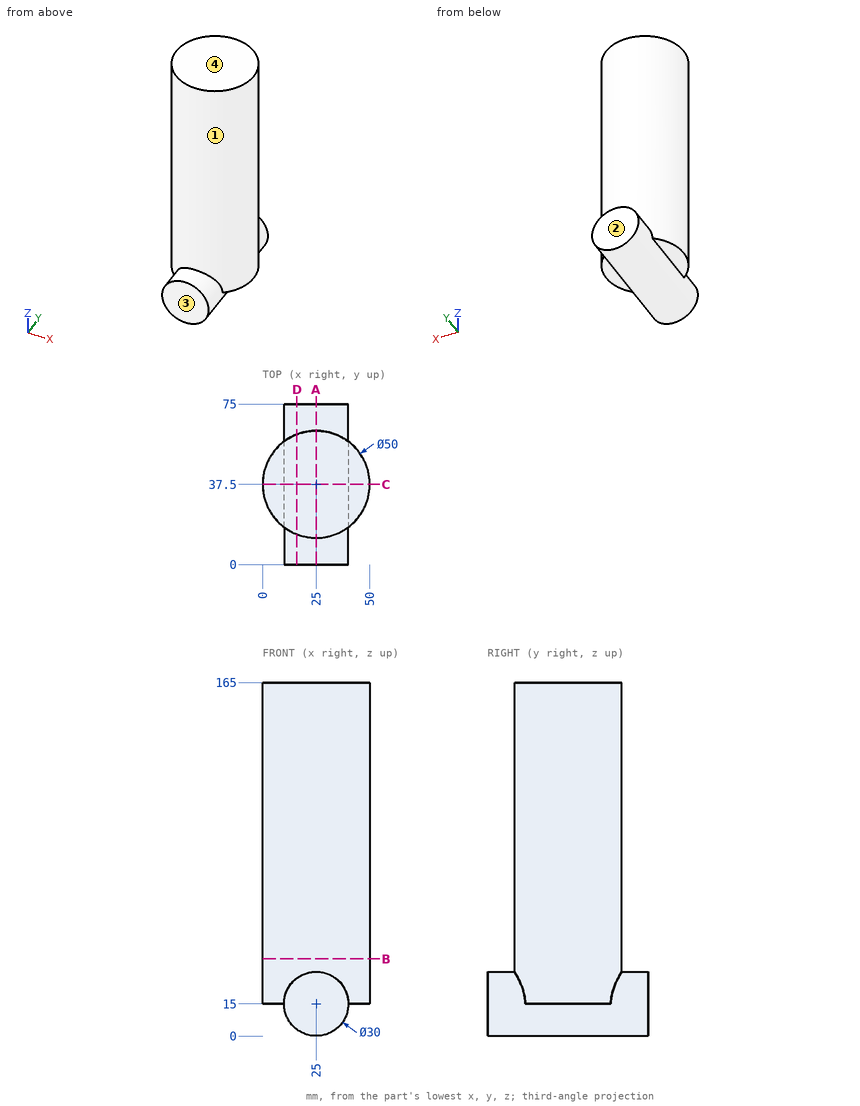
Here's the drawing with two shaded views (mm, measured from the low corner). I have some questions. Coordinates: 2 decimals unless noted, no trailing zeros. Order: outer loops, then holes, each group sorted by start corner. A loop starts at its lowest first (then second) coordinate and runs counter-clockwise, first axis right, second up.
Item 1: If we section it at A-A on x = 25: List the corners of the cut face in (y, z) for me.
Result sheet:
outline: (0, 0) - (75, 0) - (75, 30) - (62.5, 30) - (62.5, 165) - (12.5, 165) - (12.5, 30) - (0, 30) - close
Item 2: If we section it at D-D on x = 16: List the corners of the cut face in (y, z) for me, plus the area to 3 significant figures.
Result sheet:
outline: (0, 3) - (75, 3) - (75, 27) - (60.82, 27) - (60.82, 165) - (14.18, 165) - (14.18, 27) - (0, 27) - close
area: 8,240 mm2
Item 3: If we mould it in two halves opening along Y, with no side actions, what happens to the marked faces 1, 2, 3 and 4? For each: +Y half, -Y half, draft (parallel to the pull), parting line (faces both ways), or undercut.
Result sheet:
face 1: parting line
face 2: +Y half
face 3: -Y half
face 4: draft
Item 4: I need wall thicknesses on line 1 (Z direction, x = 26, y = 21.5); line 2 (Z direction, x = 26, y = 72); line 3 (Y direction, x = 33, z = 80). Which ranges of each line are inside material? Lowest first, please.
Result sheet:
line 1: z = 0.03 to 165
line 2: z = 0.03 to 29.97
line 3: y = 13.81 to 61.19
Item 5: If we section it at B-B on z = 36: List the corners of the cut face in (x, y) for me.
Result sheet:
outline: circle Ø50 at (25, 37.5)
Item 6: If we section it at C-C on y = 37.5: List the corners of the cut face in (x, z) for me, plus the area to 3 significant figures.
Result sheet:
outline: (0, 15) - (10, 15) arc R15 ccw to (40, 15) - (50, 15) - (50, 165) - (0, 165) - close
area: 7,850 mm2
Item 7: For P1, Ø1, axis at x = 41, z = 98, coming from the -Y side; P2, Ø8, axis at y = 30.5, z = 73, coming from the -X side; P3, Ø5, axis at x = 29, z = 115.5, coming from the -Y side, each with a flat end and sliding along its axis, tell me the tip position at first contact or that it passes through.
Result sheet:
P1: stops at y = 17.88
P2: stops at x = 0.18
P3: stops at y = 12.55
